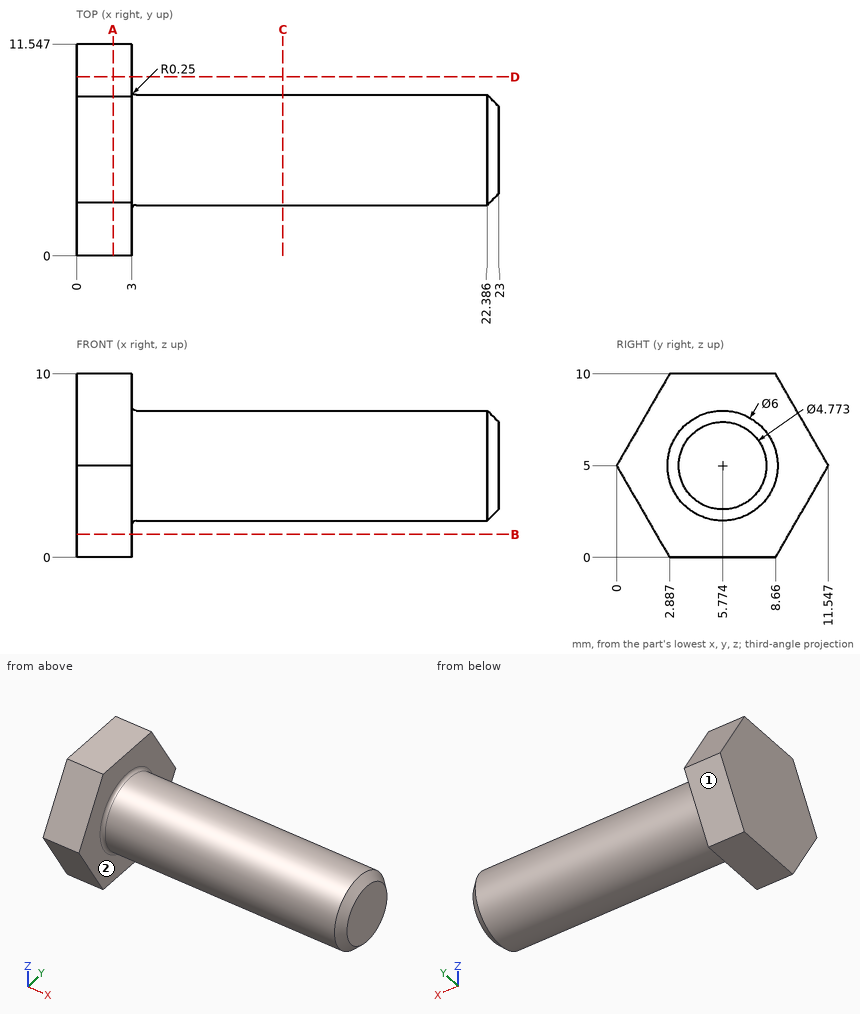
Print and shaded views of the part. All mm, measured from the part's lowest x, y and z. A direction names the side the tool comes from. Coordinates: 2 decimals unless noted, no trailing zeros. Order: outer loops, then holes, each group sorted by start corner. A loop starts at its lowest first (then second) coordinate and runs counter-clockwise, first axis right, second up. Notation, with made-up numbers: M 4.25,73.25 L 36.25,73.25 A24 cw 36.25,92.25 Z; hole C 70,-3.75 d3. An arc over 180 degrees is marked long. Answer as CSV lines item,"result".
1) Drill centre lines: L1, parallel to X at y = 9.75, z = 8; L2, parallel to Y at x = 16.25, z = 4 (1 decimal); L3, parallel to Z at x = 3.5, y = 5. Where is each one in solid material? Low to high. Write a range as from..to.
Verdict:
L1,"0..3"
L2,"2.9..8.6"
L3,"2.1..7.9"
2) Flat gauge pins, fed straight in: P1, Ø4, axis at x = 6.5, z = 3, coming from the +Y side; P2, Ø3, axis at x = 17, z = 1.5, coming from the -Y side; P3, Ø3, axis at x = 9.5, z = 7, coming from the -Y side (1 decimal). Where does each tip first touch, or does it go through?
Verdict:
P1,"y = 8.77"
P2,"y = 3.54"
P3,"y = 2.8"
3) Cut at B-B (z = 1.25). List the corners of the cut face in (x, y) (1 decimal).
Verdict:
outline,"M 0,2.2 L 3,2.2 L 3,9.4 L 0,9.4 Z"
4) Cut at A-A (x = 2). List the corners of the cut face in (y, z).
Verdict:
outline,"M 0,5 L 2.89,0 L 8.66,0 L 11.55,5 L 8.66,10 L 2.89,10 Z"
5) 3-axis set-ups, long thin cutter, end or side, ignore diameter. For the marked faces 1 and 2: which of +Z, -Z, +X, -X, +Y, -Y reach the whole face in a straight line?
Verdict:
face 1,"-Z, +X, -X, +Y"
face 2,"+X"
6) Cut at D-D (y = 9.75). List the corners of the cut face in (x, z).
Verdict:
outline,"M 0,1.89 L 3,1.89 L 3,8.11 L 0,8.11 Z"
7) Cut at C-C (x = 11.25). List the corners of the cut face in (y, z).
Verdict:
outline,"C 5.77,5 d6"
